Check sheet for the drawn part. Datum: minimum x, y, z corner. Units: mm. Give positions to 0.01 mm unless a question says otherwise; leave off trailing zeros. Order: outer loops, then holes, each group sorted by start corner. A loop starts at its lowest first (then second) coordinate and runs counter-clockwise, first axis right, second up.
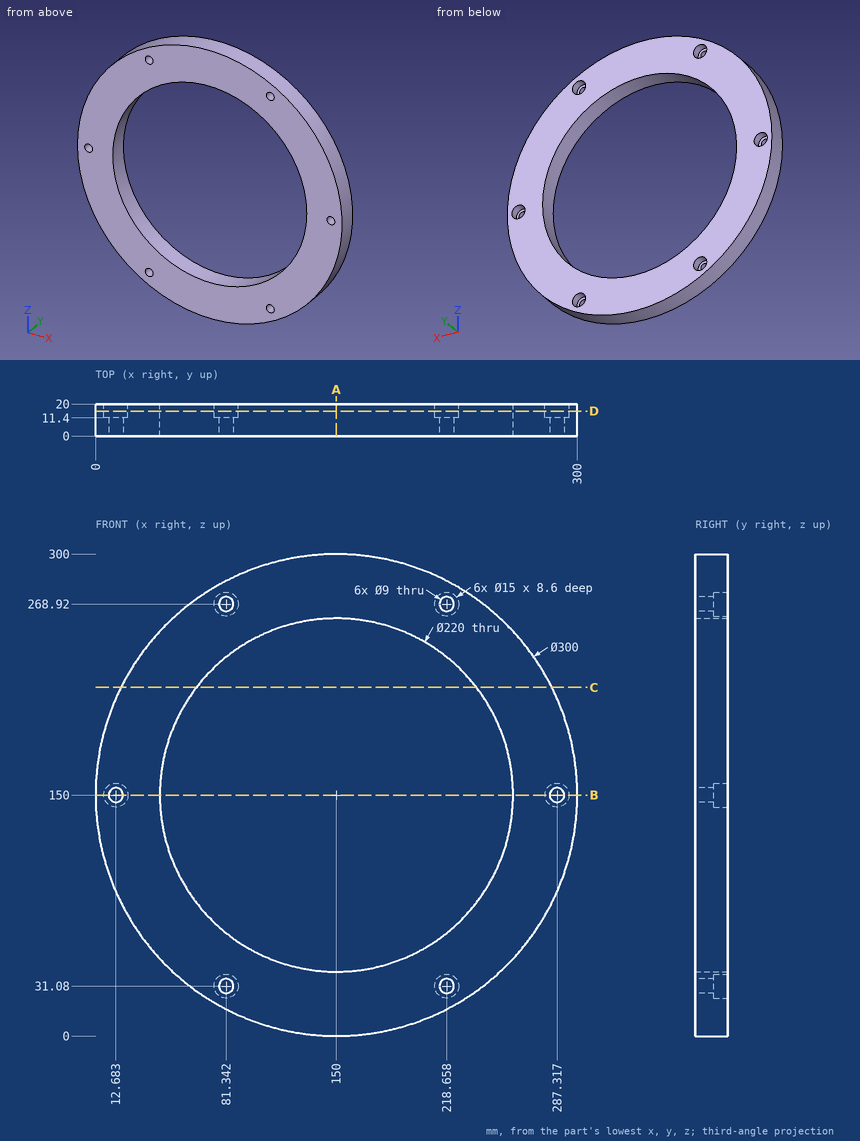
Item 1: Sectioned sample at A-A (x = 150). Enter the section's corners in (y, z).
Reported:
outline: (0, 0) - (20, 0) - (20, 40) - (0, 40) - close; (0, 260) - (20, 260) - (20, 300) - (0, 300) - close
Item 2: Sectioned sample at B-B (z = 150). Enter the section's corners in (x, y).
Reported:
outline: (0, 0) - (8.18, 0) - (8.18, 11.4) - (5.18, 11.4) - (5.18, 20) - (0, 20) - close; (17.18, 0) - (40, 0) - (40, 20) - (20.18, 20) - (20.18, 11.4) - (17.18, 11.4) - close; (260, 0) - (282.82, 0) - (282.82, 11.4) - (279.82, 11.4) - (279.82, 20) - (260, 20) - close; (291.82, 0) - (300, 0) - (300, 20) - (294.82, 20) - (294.82, 11.4) - (291.82, 11.4) - close
Item 3: Gauge pin test, flat ends, axial feed: pin 1 (16.5 mm diameter, centred on x = 220, z = 34.5, fed in from +Y); pin 2 (8 mm diameter, centred on y = 14, z = 208.5, fed in from -X); pin 3 (5 mm diameter, centred on y = 17.5, z = 206, fed in from +X) (1 decimal); pin 4 (1 mm diameter, centred on x = 85.5, y = 17, fed in from +Z). Record the tip position at first contact, or that the pin passes through.
Reported:
pin 1: stops at y = 20
pin 2: stops at x = 10.25
pin 3: stops at x = 290.1
pin 4: stops at z = 285.66
Item 4: Scan lines: L1, parallel to X at y = 12.5, z = 150; L2, parallel to Z at x = 219, y = 4.5 (1 decimal); L3, parallel to X at y = 14.5, z = 143.5 (1 decimal). Record each from-to range of solid material in increasing order.
Reported:
L1: x = 0 to 5.18, 20.18 to 40, 260 to 279.82, 294.82 to 300
L2: z = 16.8 to 26.6, 35.6 to 64.3, 235.7 to 264.4, 273.4 to 283.2
L3: x = 0.1 to 8.9, 16.4 to 40.2, 259.8 to 283.6, 291.1 to 299.9
Item 5: Sectioned sample at C-C (z = 217). Enter the section's corners in (x, y) (1 decimal), and give its area (3 significant figures).
Reported:
outline: (15.8, 0) - (62.8, 0) - (62.8, 20) - (15.8, 20) - close; (237.2, 0) - (284.2, 0) - (284.2, 20) - (237.2, 20) - close
area: 1,880 mm2
Item 6: Sectioned sample at D-D (y = 15.5). Enter the section's corners in (x, z), and give its area (3 significant figures).
Reported:
outline: circle Ø300 at (150, 150); hole circle Ø15 at (12.68, 150); hole circle Ø220 at (150, 150); hole circle Ø15 at (81.34, 31.08); hole circle Ø15 at (81.34, 268.92); hole circle Ø15 at (218.66, 31.08); hole circle Ø15 at (218.66, 268.92); hole circle Ø15 at (287.32, 150)
area: 31,600 mm2
